from build123d import *

# Parameters (mm, degrees)
SKETCH1_W           = 30
SKETCH1_H           = 100
BOSS_EXTRUDE1_DEPTH = 3.75
BOSS_EXTRUDE2_START = -0.5
BOSS_EXTRUDE2_DEPTH = 6.5


with BuildPart() as part:
    # Sketch1 → Boss-Extrude1 (new, symmetric)
    with BuildSketch(Plane(origin=(0, 0, 0), x_dir=(1, 0, 0), z_dir=(0, 1, 0))):
        with Locations((-15, 0)):
            Rectangle(SKETCH1_W, SKETCH1_H)
    extrude(amount=BOSS_EXTRUDE1_DEPTH, both=True)

    # Sketch2 → Boss-Extrude2 (add)
    with BuildSketch(Plane(origin=(0, 3.75, 0), x_dir=(1, 0, 0), z_dir=(0, 1, 0)).offset(BOSS_EXTRUDE2_START)):
        Polygon((0, 25), (15, 25.261825974), (15, -25.261825974), (0, -25), align=None)
    extrude(amount=-BOSS_EXTRUDE2_DEPTH)


solid = part.part
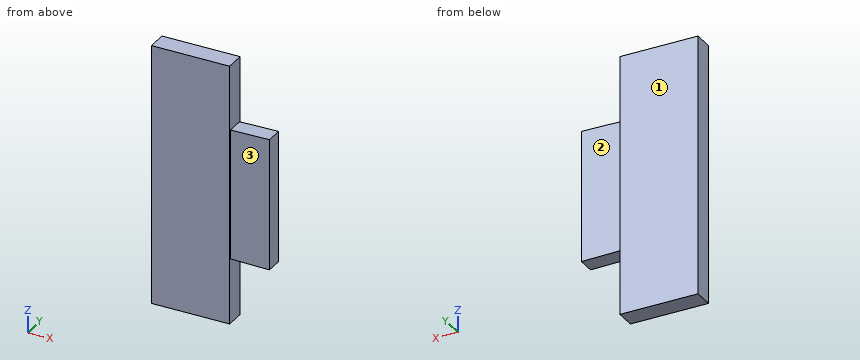
Work out the finished part from the listing and answer in its coordinate system (mm). Face numbers are marked on the shaded views. A direction names the side the tool comes from. Round coordinates to 2 decimals unless told otherwise and drop trailing zeros. Loops run counter-clockwise (first coordinate to the right, second up) from the corner with the lowest first, then second, coordinate; pieces in that order, holes last. Notation, with made-up numbers: (50, -30) - (55, -30) arc R18 cw to (55, -23) - close; hole circle Ø11 at (59.25, 36.25). An arc over 180 degrees is marked (long way). One line per item, written item: value.
Q1. Find section A-A on z = -9.5. Give the vertices of the cut face in (x, y).
Check values:
outline: (-30, -3.75) - (0, -3.75) - (0, -3.25) - (15, -3.25) - (15, 3.25) - (0, 3.25) - (0, 3.75) - (-30, 3.75) - close
Q2. Find section D-D on z = 36.5. Give the vertices of the cut face in (x, y).
Check values:
outline: (-30, -3.75) - (0, -3.75) - (0, 3.75) - (-30, 3.75) - close
Q3. Find section C-C on x = 2.5. Give the vertices of the cut face in (y, z).
Check values:
outline: (-3.25, -25.04) - (3.25, -25.04) - (3.25, 25.04) - (-3.25, 25.04) - close
Q4. Find section B-B on y = -2. Give the vertices of the cut face in (x, z), and give its area (3 significant figures).
Check values:
outline: (-30, -50) - (0, -50) - (0, -25) - (15, -25.26) - (15, 25.26) - (0, 25) - (0, 50) - (-30, 50) - close
area: 3,750 mm2
Q5. Straight lines are drawn through the part: probe 1 along Z at (x, y) = (1, -1); probe 2 along X at (y, z) = (-1, 39); probe 3 along Z at (x, y) = (4, 2.25). For each, find the intervals that lie inside material, in ascending order.
Check values:
probe 1: -25.02 to 25.02
probe 2: -30 to 0
probe 3: -25.07 to 25.07
Q6. Each of these flat-tipped pins is pushed along its axis until it touches: pin 1 Ø12 at (x, z) = (7, -3.5) entering from -Y; pin 2 Ø7.5 at (x, z) = (11, -6.5) entering from +Y. Where does it stop, or does it pass through?
Check values:
pin 1: y = -3.25
pin 2: y = 3.25
Q7. For the marked faces 1, 2 and 3, determine the directions among +Z, -Z, +X, -X, +Y, -Y from which every point of the face is accessible in a straight line to the end or side of a thin tool.
Check values:
face 1: +Z, -Z, +X, -X, +Y
face 2: +Z, -Z, +X, +Y
face 3: +Z, -Z, +X, -Y
